Read the model definition and answer for the solid it produces. Units are mm, in the model's axes. Face numbers are marked on the shaded views. A direction names the side the tool comes from. Give positions to 0.01 mm unless a question says otherwise; leave off trailing zeros. Order: outer loops, then holes, each group sorted by start corner. A loop starts at its lowest first (then second) coordinate and runs counter-clockwise, first axis right, second up.
```python
from build123d import *

# Parameters (mm, degrees)
F1_R     = 4.5
F1_R_2   = 3.175
F2_DEPTH = 4
F1_R_3   = 2.1
F3_DEPTH = 4.57
F4_DEPTH = 4.57
F5_DEPTH = 4.57
F6_DEPTH = 4.57
F1_R_4   = 2
F7_DEPTH = 15
F8_DEPTH = 15


with BuildPart() as f2:
    # F1 (on face) → F2 (new body)
    with BuildSketch(Plane.XY):
        with BuildLine():
            Line((7.709795, 12.7), (-7.690205, 12.7))
            ThreePointArc((-7.690205, 12.7), (-11.225739, 11.235534), (-12.690205, 7.7))
            Line((-12.690205, 7.7), (-12.690205, 2.634689))
            ThreePointArc((-12.690205, 2.634689), (-15.114116, -1.24147), (-19.196077, -3.3))
            ThreePointArc((-19.196077, -3.3), (-22.414634, -8.866025), (-17.490205, -13))
            Line((-17.490205, -13), (17.509795, -13))
            ThreePointArc((17.509795, -13), (22.434224, -8.866025), (19.215667, -3.3))
            ThreePointArc((19.215667, -3.3), (15.089649, -1.090359), (12.709795, 2.939881))
            Line((12.709795, 2.939881), (12.709795, 7.7))
            ThreePointArc((12.709795, 7.7), (11.245329, 11.235534), (7.709795, 12.7))
        make_face()
        with Locations((-17.490205, -8)):
            Circle(F1_R, mode=Mode.SUBTRACT)
        with BuildLine():
            ThreePointArc((-6.340205, -9.525), (-8.585269, -4.104936), (-3.165205, -6.35))
            ThreePointArc((-3.165205, -6.35), (-4.095141, -8.595064), (-6.340205, -9.525))
        make_face(mode=Mode.SUBTRACT)
        with Locations((17.509795, -8)):
            Circle(F1_R, mode=Mode.SUBTRACT)
        with Locations((6.359795, -6.35)):
            Circle(F1_R_2, mode=Mode.SUBTRACT)
        with Locations((-6.340205, 6.35)):
            Circle(F1_R_2, mode=Mode.SUBTRACT)
        with Locations((0.022334, 0.088805)):
            Circle(F1_R_2, mode=Mode.SUBTRACT)
        with Locations((6.359795, 6.35)):
            Circle(F1_R_2, mode=Mode.SUBTRACT)
    extrude(amount=F2_DEPTH)

    # F1 (on face) → F3 (join)
    with BuildSketch(Plane.XY):
        with Locations((-6.340205, 6.35)):
            Circle(F1_R_2)
        with Locations((-6.340205, 6.35)):
            Circle(F1_R_3, mode=Mode.SUBTRACT)
    extrude(amount=F3_DEPTH)

    # F1 (on face) → F4 (join)
    with BuildSketch(Plane.XY):
        with Locations((6.359795, 6.35)):
            Circle(F1_R_2)
        with Locations((6.359795, 6.35)):
            Circle(F1_R_3, mode=Mode.SUBTRACT)
    extrude(amount=F4_DEPTH)

    # F1 (on face) → F5 (join)
    with BuildSketch(Plane.XY):
        with Locations((6.359795, -6.35)):
            Circle(F1_R_2)
        with Locations((6.359795, -6.35)):
            Circle(F1_R_3, mode=Mode.SUBTRACT)
    extrude(amount=F5_DEPTH)

    # F1 (on face) → F6 (join)
    with BuildSketch(Plane.XY):
        with BuildLine():
            ThreePointArc((-6.340205, -9.525), (-4.095141, -8.595064), (-3.165205, -6.35))
            ThreePointArc((-3.165205, -6.35), (-8.585269, -4.104936), (-6.340205, -9.525))
        make_face()
        with Locations((-6.340205, -6.35)):
            Circle(F1_R_3, mode=Mode.SUBTRACT)
    extrude(amount=F6_DEPTH)

    # F1 (on face) → F7 (join)
    with BuildSketch(Plane.XY):
        with Locations((-17.490205, -8)):
            Circle(F1_R)
        with Locations((-17.490205, -8)):
            Circle(F1_R_4, mode=Mode.SUBTRACT)
    extrude(amount=F7_DEPTH)

    # F1 (on face) → F8 (join)
    with BuildSketch(Plane.XY):
        with Locations((17.509795, -8)):
            Circle(F1_R)
        with Locations((17.509795, -8)):
            Circle(F1_R_4, mode=Mode.SUBTRACT)
    extrude(amount=F8_DEPTH)


solid = f2.part
```
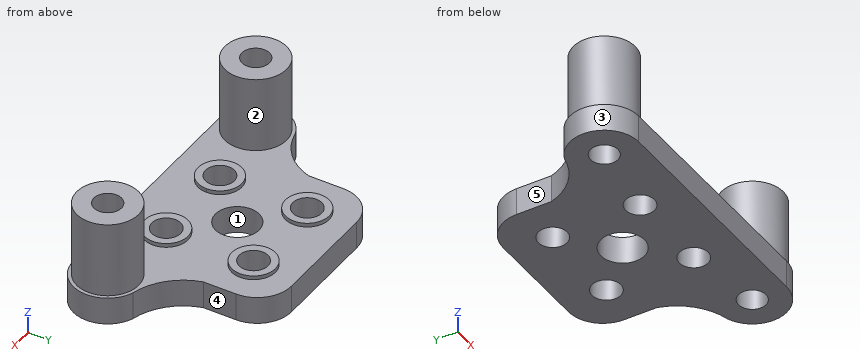
1) Consider L1, parallel to Z at x = -3.5, y = -7.25; L2, parallel to Z at x = -3, y = -6.25; L3, parallel to Y at x = 19, z = 13.5. Determine where each line is inside the solid, lowest interval first.
Final values:
L1: z = 0 to 4.57
L2: z = 0 to 4
L3: y = -12.25 to -9.33, -6.67 to -3.75
2) Given pin 1 (1.5 mm diameter, centred on y = -8.5, z = 6, fed in from -X); pin 2 (2 mm diameter, centred on y = 6, z = 1, fed in from +X); pin 3 (3.5 mm diameter, centred on x = -6.34, y = 6.35, fed in from +Z); pin 4 (3 mm diameter, centred on y = 4, z = 2.5, fed in from -X), each flat-ended and moving along its own axis, determine where each tip first touches the part or whether it passes through.
Final values:
pin 1: stops at x = -21.99
pin 2: stops at x = 12.71
pin 3: passes through
pin 4: stops at x = -12.73
3) The part is cut by section A-A on y = 6.35. Determine the outline of the cut face in (x, z), and give its area (3 significant figures).
Final values:
outline: (-12.69, 0) - (-8.44, 0) - (-8.44, 4.57) - (-9.52, 4.57) - (-9.52, 4) - (-12.69, 4) - close; (-4.24, 0) - (4.26, 0) - (4.26, 4.57) - (3.18, 4.57) - (3.18, 4) - (-3.17, 4) - (-3.17, 4.57) - (-4.24, 4.57) - close; (8.46, 0) - (12.71, 0) - (12.71, 4) - (9.53, 4) - (9.53, 4.57) - (8.46, 4.57) - close
area: 70.5 mm2
4) A tool of negligible diameter and unlimited length cuts with its end or side. For the marked faces 1, 2, 3, 4 and 5, from which of +Z, -Z, +X, -X, +Y, -Y can it reach the whole face along a straight path? Write none if from no direction.
Final values:
face 1: +Z, -Z
face 2: +Z
face 3: +Z, -Z, -X
face 4: +Z, -Z, +X, +Y
face 5: +Z, -Z, -X, +Y
5) The part is cut by section B-B on x = 6.5. Determine the outline of the cut face in (y, z), and give its area (3 significant figures).
Final values:
outline: (-13, 0) - (-8.45, 0) - (-8.45, 4.57) - (-9.52, 4.57) - (-9.52, 4) - (-13, 4) - close; (-4.25, 0) - (4.25, 0) - (4.25, 4.57) - (3.18, 4.57) - (3.18, 4) - (-3.18, 4) - (-3.18, 4.57) - (-4.25, 4.57) - close; (8.45, 0) - (12.7, 0) - (12.7, 4) - (9.52, 4) - (9.52, 4.57) - (8.45, 4.57) - close
area: 71.7 mm2
6) The part is cut by section D-D on z = 5.25. Determine the outline of the cut face in (x, y).
Final values:
outline: circle Ø9 at (-17.49, -8); circle Ø9 at (17.51, -8); hole circle Ø4 at (-17.49, -8); hole circle Ø4 at (17.51, -8)
7) The part is cut by section C-C on x = -16. Determine the outline of the cut face in (y, z), and give its area (3 significant figures).
Final values:
outline: (-13, 0) - (-9.33, 0) - (-9.33, 15) - (-12.25, 15) - (-12.25, 4) - (-13, 4) - close; (-6.67, 0) - (-1.95, 0) - (-1.95, 4) - (-3.75, 4) - (-3.75, 15) - (-6.67, 15) - close
area: 97.6 mm2
